Can you work these out from the model? Positions are in its coordinate system, mm. Round coordinates to 2 decimals unless told otherwise and drop trailing zeros. Order: outer loops, then holes, each group sorted by start corner. A loop starts at its lowest first (then second) coordinate and runs counter-clockwise, first axis right, second up.
from build123d import *

# Parameters (mm, degrees)
F0_W     = 101.6
F0_H     = 254
F1_DEPTH = 6.35
F3_D     = 7.9375
F5_D     = 7.9375


with BuildPart() as f1:
    # F0 (on Front) → F1 (new body)
    with BuildSketch(Plane.XZ):
        with Locations((50.8, 127)):
            Rectangle(F0_W, F0_H)
    extrude(amount=F1_DEPTH)

    # F3 (through all)
    with Locations(Plane.XZ.offset(6.35)):
        with Locations((83.376482, 57.15), (83.376482, 196.85)):
            Hole(F3_D / 2)

    # F5 (through all)
    with Locations(Plane.XZ.offset(6.35)):
        with Locations((14.246169, 76.2), (14.246169, 177.8)):
            Hole(F5_D / 2)


solid = f1.part
(1) I want a section at A-A, the plane z = 196.85. List the corners of the cut face in (x, y) for me.
(2) If we mould it in two halves opening along X, with no side actions, what happens to faces 1 (the face through (50, -3, 0)), 2 (the face through (0, -3, 125)), 3 (the face through (86.5, -3.1, 54.7))? For each: pulls with the +X half, pulls with the -X half, needs draft (parallel to the pull), parting line crosses it, or undercut.
(3) Please list where these lines run through material, in increasing order: probe 1 along Z at (x, y) = (14.5, -1.25); probe 2 along Z at (x, y) = (12.5, -1); probe 3 along X at (y, z) = (-1.25, 54).
Ans:
1. outline: (0, -6.35) - (79.41, -6.35) - (79.41, 0) - (0, 0) - close; (87.35, -6.35) - (101.6, -6.35) - (101.6, 0) - (87.35, 0) - close
2. face 1: needs draft
2. face 2: pulls with the -X half
2. face 3: undercut
3. probe 1: z = 0 to 72.24, 80.16 to 173.84, 181.76 to 254
3. probe 2: z = 0 to 72.64, 79.76 to 174.24, 181.36 to 254
3. probe 3: x = 0 to 80.96, 85.79 to 101.6
